```python
from build123d import *

# Parameters (mm, degrees)
F0_R     = 2.25
F1_DEPTH = 2.5
F2_R     = 2
F3_DEPTH = 15
F4_W     = 9
F4_H     = 33
F5_DEPTH = 5


with BuildPart() as f1:
    # F0 (on Top) → F1 (new body)
    with BuildSketch(Plane.XY):
        with BuildLine():
            ThreePointArc((19.25, 32.5), (15.40901, 34.09099), (17, 30.25))
            ThreePointArc((17, 30.25), (18.59099, 30.90901), (19.25, 32.5))
        make_face()
        Polygon((12.5, 19), (12.5, 0), (22.5, 0), (22.5, 38), (12.5, 38), align=None)
        with Locations((17, 5.5)):
            Circle(F0_R, mode=Mode.SUBTRACT)
        with BuildLine():
            ThreePointArc((19.25, 32.5), (18.59099, 30.90901), (17, 30.25))
            ThreePointArc((17, 30.25), (15.40901, 34.09099), (19.25, 32.5))
        make_face(mode=Mode.SUBTRACT)
    extrude(amount=F1_DEPTH)

    # F2 (on Top) → F3 (join)
    with BuildSketch(Plane.XY):
        with BuildLine():
            ThreePointArc((7.5, 28.25), (4.085786, 29.664214), (5.5, 26.25))
            ThreePointArc((5.5, 26.25), (6.914214, 26.835786), (7.5, 28.25))
        make_face()
        Polygon((1.5, 19), (1.5, 0), (12.5, 0), (12.5, 38), (1.5, 38), align=None)
        with Locations((5.5, 9.75)):
            Circle(F2_R, mode=Mode.SUBTRACT)
        with BuildLine():
            ThreePointArc((7.5, 28.25), (6.914214, 26.835786), (5.5, 26.25))
            ThreePointArc((5.5, 26.25), (4.085786, 29.664214), (7.5, 28.25))
        make_face(mode=Mode.SUBTRACT)
    extrude(amount=F3_DEPTH)

    # F4 (on Top) → F5 (cut)
    with BuildSketch(Plane.XY):
        with Locations((6, 19)):
            Rectangle(F4_W, F4_H)
    extrude(amount=F5_DEPTH, mode=Mode.SUBTRACT)


solid = f1.part
```
The listing builds one solid part. Answer for the finished solid, in the listing's coordinates (mm). A direction names the side the tool comes from. Round coordinates to 2 decimals unless told otherwise and drop trailing zeros. Loops run counter-clockwise (first coordinate to the right, second up) from the corner with the lowest first, then second, coordinate; pieces in that order, holes last.
1) For faces 1 (the face through (5.24, 11.733, 9.93)), 2 (the face through (12.5, 19, 9)), 3 (the face through (6, 19, 5)), determine the directions among +Z, -Z, +X, -X, +Y, -Y from which every point of the face is accessible in a straight line to the end or side of a thin tool.
Outcome:
face 1: +Z, -Z
face 2: +Z, +X, +Y, -Y
face 3: -Z, -X
2) A cutting plane is placed at A-A on y = 5.5. Determine the outline of the cut face in (x, z).
Outcome:
outline: (1.5, 5) - (10.5, 5) - (10.5, 0) - (14.75, 0) - (14.75, 2.5) - (12.5, 2.5) - (12.5, 15) - (1.5, 15) - close; (19.25, 0) - (22.5, 0) - (22.5, 2.5) - (19.25, 2.5) - close
3) For a pull along Y with two mould halves and no side action, classify faces 4 (the face through (10, 0, 6)), 5 (the face through (10.5, 19, 2)), 6 (the face through (17, 19, 2.5)) as released by +Y, released by -Y, zero draft, split by the parting line, or undercut.
Outcome:
face 4: released by -Y
face 5: undercut
face 6: zero draft
4) Given P1, Ø2, axis at y = 24.5, z = 3.5, coming from the -X side; P2, Ø3, axis at x = 17.5, y = 28.5, coming from the +Z side; P3, Ø3.5, axis at x = 17, y = 32.5, coming from the -Z side, each flat-ended and moving along its own axis, determine where each tip first touches the part or whether it passes through.
Outcome:
P1: stops at x = 10.5
P2: stops at z = 2.5
P3: passes through
5) Consider line 1 (Y direction, x = 17, z = 0.8); line 2 (X direction, y = 32.5, z = 1.6); line 3 (Y direction, x = 5.5, z = 10.5). Determine where each line is inside the solid, lowest interval first.
Outcome:
line 1: y = 0 to 3.25, 7.75 to 30.25, 34.75 to 38
line 2: x = 10.5 to 14.75, 19.25 to 22.5
line 3: y = 0 to 7.75, 11.75 to 26.25, 30.25 to 38
6) A cutting plane is placed at C-C on x = 17.75. Determine the outline of the cut face in (y, z).
Outcome:
outline: (0, 0) - (3.38, 0) - (3.38, 2.5) - (0, 2.5) - close; (7.62, 0) - (30.38, 0) - (30.38, 2.5) - (7.62, 2.5) - close; (34.62, 0) - (38, 0) - (38, 2.5) - (34.62, 2.5) - close
7) A cutting plane is placed at D-D on x = 9.25. Determine the outline of the cut face in (y, z), plus the area to 3 significant figures.
Outcome:
outline: (0, 0) - (2.5, 0) - (2.5, 5) - (35.5, 5) - (35.5, 0) - (38, 0) - (38, 15) - (0, 15) - close
area: 405 mm2
8) A cutting plane is placed at B-B on z = 8. Determine the outline of the cut face in (x, y).
Outcome:
outline: (1.5, 0) - (12.5, 0) - (12.5, 38) - (1.5, 38) - close; hole circle Ø4 at (5.5, 9.75); hole (5.5, 26.25) arc R2 ccw to (7.5, 28.25) arc R2 ccw (long way) to start
